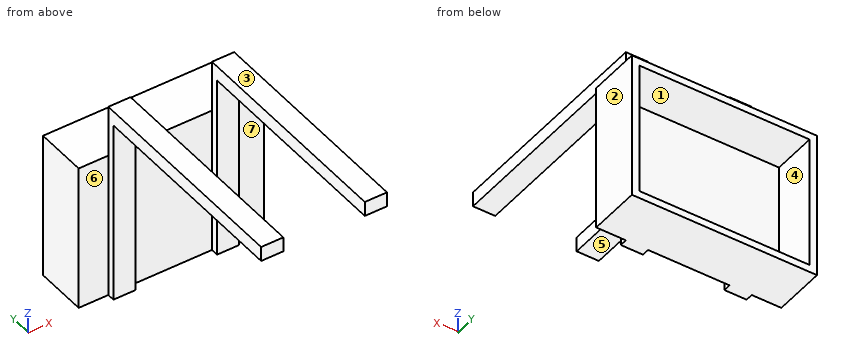
```python
from build123d import *

# Parameters (mm, degrees)
CROQUIS1_W              = 250
CROQUIS1_H              = 200
SALIENTE_EXTRUIR1_DEPTH = 10
CROQUIS2_W              = 250
CROQUIS2_H              = 200
CROQUIS2_W_2            = 230
CROQUIS2_H_2            = 180
SALIENTE_EXTRUIR2_DEPTH = 60
CROQUIS3_W              = 30
CROQUIS3_H              = 270
SALIENTE_EXTRUIR3_DEPTH = 10
CROQUIS4_W              = 30
CROQUIS4_H              = 20
SALIENTE_EXTRUIR4_DEPTH = 290


with BuildPart() as part:
    # Croquis1 → Saliente-Extruir1 (new body)
    with BuildSketch(Plane(origin=(0, 0, 0), x_dir=(1, 0, 0), z_dir=(0, 1, 0))):
        Rectangle(CROQUIS1_W, CROQUIS1_H)
    extrude(amount=SALIENTE_EXTRUIR1_DEPTH)

    # Croquis2 → Saliente-Extruir2 (add)
    with BuildSketch(Plane(origin=(0, 10, 0), x_dir=(1, 0, 0), z_dir=(0, 1, 0))):
        Rectangle(CROQUIS2_W, CROQUIS2_H)
        Rectangle(CROQUIS2_W_2, CROQUIS2_H_2, mode=Mode.SUBTRACT)
    extrude(amount=SALIENTE_EXTRUIR2_DEPTH)

    # Croquis3 → Saliente-Extruir3 (add)
    with BuildSketch(Plane.XZ):
        with Locations((-70, 35)):
            Rectangle(CROQUIS3_W, CROQUIS3_H)
        with Locations((70, 35)):
            Rectangle(CROQUIS3_W, CROQUIS3_H)
    extrude(amount=SALIENTE_EXTRUIR3_DEPTH)

    # Croquis4 → Saliente-Extruir4 (add)
    with BuildSketch(Plane.XZ.offset(10)):
        with Locations((-70, 160)):
            Rectangle(CROQUIS4_W, CROQUIS4_H)
        with Locations((70, 160)):
            Rectangle(CROQUIS4_W, CROQUIS4_H)
    extrude(amount=SALIENTE_EXTRUIR4_DEPTH)


solid = part.part
```
Verification items for the finished model (mm, model axes). Face numbers are marked on the shaded views. A direction names the side the tool comes from. Coordinates: 2 decimals unless noted, no trailing zeros. Loops run counter-clockwise (first coordinate to the right, second up) from the corner with the lowest first, then second, coordinate; pieces in that order, holes last. Notation, with made-up numbers: (41, -29.75) - (59, -29.75) arc R18 ccw to (59, -19.75) - close; hole circle Ø4 at (44.25, 73.25). An arc over 180 degrees is marked (long way). Put each result on its own line as item: value.
Item 1: Set-up check for the marked faces 5, 6 and 7: record each of +Z, -Z, +X, -X, +Y, -Y from which the full face is reachable in a straight line by a thin tool's end or side.
Conclusion:
face 5: -Z, +X, -X, -Y
face 6: +Z, -Z, -X, -Y
face 7: +Z, -Z, +X, -Y
Item 2: Section check C-C (z = -49). Enter the section's corners in (x, y), then the cut area to 3 significant figures.
Conclusion:
outline: (-125, 0) - (-85, 0) - (-85, -10) - (-55, -10) - (-55, 0) - (55, 0) - (55, -10) - (85, -10) - (85, 0) - (125, 0) - (125, 70) - (115, 70) - (115, 10) - (-115, 10) - (-115, 70) - (-125, 70) - close
area: 4,300 mm2
Item 3: Section check A-A (y = -162). Enter the section's corners in (x, z), then the cut area to 3 significant figures.
Conclusion:
outline: (-85, 150) - (-55, 150) - (-55, 170) - (-85, 170) - close; (55, 150) - (85, 150) - (85, 170) - (55, 170) - close
area: 1,200 mm2
Item 4: Gauge pin test, flat ends, axial feed: pin 1 Ø15 at (x, z) = (-74.5, 143.5) entering from +Y; pin 2 Ø3 at (x, y) = (-1.5, 21) entering from +Z; pin 3 Ø12 at (x, z) = (-111.5, 34.5) entering from -Y. Record the tip position at first contact, or that the pin passes through.
Conclusion:
pin 1: stops at y = 0
pin 2: stops at z = 100
pin 3: stops at y = 0
Item 5: Section check D-D (x = 60). Enter the section's corners in (y, z), then the cut area to 3 significant figures.
Conclusion:
outline: (-300, 150) - (-10, 150) - (-10, -100) - (70, -100) - (70, -90) - (10, -90) - (10, 90) - (70, 90) - (70, 100) - (0, 100) - (0, 170) - (-300, 170) - close
area: 11,700 mm2
Item 6: Section check B-B (x = -2.5). Enter the section's corners in (y, z), then the cut area to 3 significant figures.
Conclusion:
outline: (0, -100) - (70, -100) - (70, -90) - (10, -90) - (10, 90) - (70, 90) - (70, 100) - (0, 100) - close
area: 3,200 mm2
Item 7: Scan lines: line 1 along X through (y, z) = (36.5, 8.5); line 2 along Z through (x, y) = (100.5, 30); line 3 along X through (y, z) = (-2, -40). Record each from-to range of solid material in increasing order.
Conclusion:
line 1: x = -125 to -115, 115 to 125
line 2: z = -100 to -90, 90 to 100
line 3: x = -85 to -55, 55 to 85
Item 8: Draft check along Z on the marked faces 1, 2, 3 and 4. Enter one of: pulls with the +Z half, pulls with the -Z half, needs draft (parallel to the pull), parting line crosses it, or undercut.
Conclusion:
face 1: undercut
face 2: needs draft
face 3: pulls with the +Z half
face 4: undercut
